```python
from build123d import *

# Parameters (mm, degrees)
BOSS_EXTRUDE1_DEPTH     = 60
BOSS_EXTRUDE2_DEPTH     = 25
BOSS_EXTRUDE3_DEPTH     = 25
BOSS_EXTRUDE4_DEPTH     = 25
CUT_EXTRUDE2_DEPTH      = 191.91883092
CUT_EXTRUDE2_DEPTH_BACK = 191.91883092
SKETCH6_R               = 15
CUT_EXTRUDE3_DEPTH      = 183.551362635
CUT_EXTRUDE3_DEPTH_BACK = 183.551362635
SKETCH7_R               = 15


with BuildPart() as part:
    # Sketch1 → Boss-Extrude1 (new body)
    with BuildSketch(Plane.XY):
        Polygon((0, 0), (60, 0), (60, -25), (135, -25), (135, -50), (60, -50), (60, -75), (0, -75), (0, -50), (35, -50), (35, -25), (0, -25), align=None)
    extrude(amount=BOSS_EXTRUDE1_DEPTH)

    # Sketch3 → Boss-Extrude2 (add)
    with BuildSketch(Plane(origin=(0, 0, 0), x_dir=(1, 0, 0), z_dir=(0, 1, 0))):
        with BuildLine():
            Line((0, 0), (0, -60))
            ThreePointArc((0, -60), (-30, -30), (0, 0))
        make_face()
    extrude(amount=-BOSS_EXTRUDE2_DEPTH)

    # Sketch4 → Boss-Extrude3 (add)
    with BuildSketch(Plane(origin=(0, -50, 0), x_dir=(1, 0, 0), z_dir=(0, 1, 0))):
        with BuildLine():
            Line((0, 0), (0, -60))
            ThreePointArc((0, -60), (-30, -30), (0, 0))
        make_face()
    extrude(amount=-BOSS_EXTRUDE3_DEPTH)

    # Sketch5 → Boss-Extrude4 (add)
    with BuildSketch(Plane(origin=(0, -25, 0), x_dir=(1, 0, 0), z_dir=(0, 1, 0))):
        with BuildLine():
            Line((135, 0), (135, -60))
            ThreePointArc((135, -60), (165, -30), (135, 0))
        make_face()
    extrude(amount=-BOSS_EXTRUDE4_DEPTH)

    # Sketch6 → Cut-Extrude2 (cut, two sides: drawn at the far end of the back side and taken through both)
    with BuildSketch(Plane(origin=(0, 0, 0), x_dir=(1, 0, 0), z_dir=(0, 1, 0)).offset(-CUT_EXTRUDE2_DEPTH_BACK)):
        with Locations(Location((0, -30, 0), (0, 0, 270))):
            Circle(SKETCH6_R)
    extrude(amount=CUT_EXTRUDE2_DEPTH + CUT_EXTRUDE2_DEPTH_BACK, mode=Mode.SUBTRACT)

    # Sketch7 → Cut-Extrude3 (cut, two sides: drawn at the far end of the back side and taken through both)
    with BuildSketch(Plane(origin=(0, -25, 0), x_dir=(1, 0, 0), z_dir=(0, 1, 0)).offset(-CUT_EXTRUDE3_DEPTH_BACK)):
        with Locations(Location((135, -30, 0), (0, 0, 180))):
            Circle(SKETCH7_R)
    extrude(amount=CUT_EXTRUDE3_DEPTH + CUT_EXTRUDE3_DEPTH_BACK, mode=Mode.SUBTRACT)


solid = part.part
```
Design review of the part built by this model. Coordinates are the model's own, in mm. A direction names the side the tool comes from. Give positions to 0.01 mm unless a question says otherwise; leave off trailing zeros. Loops run counter-clockwise (first coordinate to the right, second up) from the corner with the lowest first, then second, coordinate; pieces in that order, holes last. Notation, with made-up numbers: (59, -2) -> (77, -2) arc R12 ccw to (77, 5) -> close; hole circle Ø3 at (59, -32). An arc over 180 degrees is marked (long way). Write each question's results on one line, items separated by ' | '.
Q1. Take a section at C-C, the plane x = 123.5. Write out the cut boundary in (y, z).
Reply:
outline: (-50, 0) -> (-25, 0) -> (-25, 20.37) -> (-50, 20.37) -> close; (-50, 39.63) -> (-25, 39.63) -> (-25, 60) -> (-50, 60) -> close
Q2. Wall thickness on L1, parallel to Z at x = 135, y = -38.75; L2, parallel to Y at x = 25, z = 39; L3, parallel to X at y = -44, z = 30: over which ranges is each line inside the solid? List them lowest first.
Reply:
L1: z = 0 to 15, 45 to 60 | L2: y = -75 to -50, -25 to 0 | L3: x = 35 to 120, 150 to 165
Q3. Take a section at D-D, the plane z = 40. Write out the cut boundary in (x, y), plus the area to 3 significant figures.
Reply:
outline: (-28.28, -75) -> (-11.18, -75) -> (-11.18, -50) -> (-28.28, -50) -> close; (-28.28, -25) -> (-11.18, -25) -> (-11.18, 0) -> (-28.28, 0) -> close; (11.18, -75) -> (60, -75) -> (60, -50) -> (123.82, -50) -> (123.82, -25) -> (60, -25) -> (60, 0) -> (11.18, 0) -> (11.18, -25) -> (35, -25) -> (35, -50) -> (11.18, -50) -> close; (146.18, -50) -> (163.28, -50) -> (163.28, -25) -> (146.18, -25) -> close | area: 5,940 mm²
Q4. Take a section at B-B, the plane y = -18. Write out the cut boundary in (x, z), plus the area to 3 significant figures.
Reply:
outline: (0, 0) -> (60, 0) -> (60, 60) -> (0, 60) arc R30 ccw to start; hole circle Ø30 at (0, 30) | area: 4,310 mm²
Q5. Machinability: for faces 5 (the face through (-29.993, -62.325, 30.66)), 6 (the face through (100, -25, 30)), 7 (the face through (100, -50, 30)), 8 (the face through (12.65, -12.68, 38.06)), 9 (the face through (17, -50, 30)), which of the approach directions +Z, -Z, +X, -X, +Y, -Y give a long, thin tool a straight path to every point of the face, cutting with its end or side? Answer none if there is none.
Reply:
face 5: -X, +Y, -Y | face 6: +Z, -Z, +X, +Y | face 7: +Z, -Z, +X, -Y | face 8: +Y, -Y | face 9: +Z, -Z, -X
Q6. The part is to be moulded in two halves that separate along X. For faces 1 (the face through (-29.993, -12.325, 30.66)), 2 (the face through (12.65, -62.68, 38.06)), 3 (the face through (60, -62, 30)), 4 (the face through (26, -75, 30)), say which applies: +X half, -X half, draft (parallel to the pull), parting line (faces both ways), or undercut.
Reply:
face 1: -X half | face 2: undercut | face 3: +X half | face 4: draft
Q7. For pin 1 Ø2 at (y, z) = (-8, 53) entering from -X; pin 2 Ø7.5 at (y, z) = (-10, 42.5) entering from +X; pin 3 Ø10 at (x, z) = (104.5, 53.5) entering from +Y, all flat-tipped, find the tip position at first contact; note any pin that passes through.
Reply:
pin 1: stops at x = -20.4 | pin 2: stops at x = 60 | pin 3: stops at y = -25
Q8. Take a section at A-A, the plane z = 30. Write out the cut boundary in (x, y), plus the area to 3 significant figures.
Reply:
outline: (-30, -75) -> (-15, -75) -> (-15, -50) -> (-30, -50) -> close; (-30, -25) -> (-15, -25) -> (-15, 0) -> (-30, 0) -> close; (15, -75) -> (60, -75) -> (60, -50) -> (120, -50) -> (120, -25) -> (60, -25) -> (60, 0) -> (15, 0) -> (15, -25) -> (35, -25) -> (35, -50) -> (15, -50) -> close; (150, -50) -> (165, -50) -> (165, -25) -> (150, -25) -> close | area: 5,500 mm²
